Autodesk Inventor part; units mm, degrees
ref_plane "Work Plane1" through (215.9, 0, 0) normal (1, 0, 0) x (0, 0, -1)
ref_plane "YZ Plane" through (0, 0, 0) normal (1, 0, 0) x (0, 1, 0)
ref_plane "XZ Plane" through (0, 0, 0) normal (0, 1, 0) x (-1, 0, 0)
sketch "Sketch1" plane through (0, 0, 0) normal (1, 0, 0) x (0, 1, 0)
  line L0 (0, -50.8) -> (0, 50.8) construction
  line L1 (19.05, -50.8) -> (19.05, 50.8)
  line L2 (-19.05, 50.8) -> (-19.05, -50.8)
  arc A0 (-19.05, -50.8) -> (19.05, -50.8) centre (0, -50.8) ccw
  arc A1 (19.05, 50.8) -> (-19.05, 50.8) centre (0, 50.8) ccw
  circle A2 centre (0, 50.8) radius 14.2875
  circle A3 centre (0, -50.8) radius 6.35
  point P0 (0, 0)
  dimension "d0" = 50.8
  dimension "d1" = 38.1
  dimension "d2" = 28.575
  dimension "d12" = 12.7
extrude "Extrusion1" add sketch "Sketch1" along normal blind 7.9375
sketch "Sketch2" plane through (7.9375, 0, 0) normal (1, 0, 0) x (0, 0, -1)
  circle A0 centre (0, 0) radius 12.7
  circle A1 centre (0, 0) radius 15.875
  dimension "d5" = 25.4
  dimension "d6" = 31.75
extrude "Extrusion2" add sketch "Sketch2" along normal blind 207.9625
ref_plane "Work Plane1" through (215.9, 0, 0) normal (1, 0, 0) x (0, 0, -1)
sketch "Sketch3" plane through (215.9, 0, 0) normal (1, 0, 0) x (0, 0, -1)
  arc A0 (-50.8, 19.05) -> (-50.8, -19.05) centre (-50.8, 0) ccw
  circle A1 centre (-50.8, 0) radius 14.2875
  line L0 (50.8, 19.05) -> (-50.8, 19.05)
  arc A2 (50.8, -19.05) -> (50.8, 19.05) centre (50.8, 0) ccw
  line L1 (-50.8, -19.05) -> (50.8, -19.05)
  circle A3 centre (50.8, 0) radius 6.35
  point P0 (0, 0)
  dimension "d13" = 101.6
extrude "Extrusion3" add sketch "Sketch3" along normal blind 7.9375
properties part number "toggle" material "Steel, Wrought"
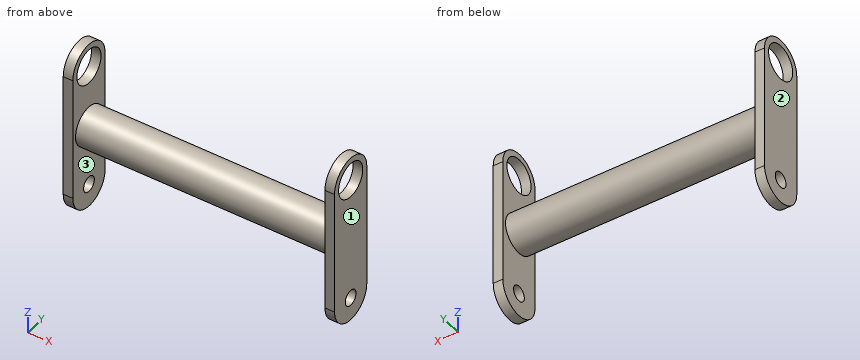
Design review of the part built by this model. Coordinates are the model's own, in mm. Face numbers are marked on the shaded views. Round coordinates to 2 decimals unless told otherwise and drop trailing zeros. Order: outer loops, then holes, each group sorted by start corner. A loop starts at its lowest first (then second) coordinate and runs counter-clockwise, first axis right, second up. Notation, with made-up numbers: (17.5, -2.5) - (64.5, -2.5) arc R10 cw to (64.5, 4.5) - close; hole circle Ø1 at (32, 78.5). An arc over 180 degrees is marked (long way). Return JSON: item names as keys, results as strings.
Q1. The part is to be moulded in two halves that separate along X. For the marked faces 1, 2 and 3, say which applies: pulls with the +X half, pulls with the -X half, needs draft (parallel to the pull), parting line crosses it, or undercut.
Computed values:
{"face 1": "pulls with the +X half", "face 2": "pulls with the -X half", "face 3": "undercut"}
Q2. Consider section A-A on y = 0. Give the number of separate pieces and of enclosed holes in the cut face, plus the area to 3 significant figures.
Computed values:
{"separate pieces": "5", "enclosed holes": "1", "area": "2,880 mm2"}
Q3. For pin 1 Ø1.5 at (x, y) = (167.5, -7.5) entering from -Z; pin 2 Ø8 at (x, y) = (46, 8.5) entering from +Z; pin 3 Ø8 at (x, y) = (28.5, -5.5) entering from -Z, all flat-tipped, find the tip position at first contact; note any pin that passes through.
Computed values:
{"pin 1": "stops at z = -14.37", "pin 2": "stops at z = 15.22", "pin 3": "stops at z = -15.8"}
Q4. Wall thickness on L1, parallel to Z at x = 5, y = 0; L2, parallel to X at y = -11, z = -63.5; L3, parallel to Y at x = 161, z = 0 (3 decimals): over which ranges is each line inside the solid? List them lowest first. Write a range as [from, to].
Computed values:
{"L1": "z = [-69.85, -57.15], [-44.45, 36.51], [65.09, 69.85]", "L2": "x = [0, 7.94], [215.9, 223.84]", "L3": "y = [-15.875, -12.7], [12.7, 15.875]"}
Q5. Consider section B-B on z = -27.5. Write out the cut boundary in (x, y).
Computed values:
{"outline": "(0, -19.05) - (7.94, -19.05) - (7.94, 19.05) - (0, 19.05) - close; (215.9, -19.05) - (223.84, -19.05) - (223.84, 19.05) - (215.9, 19.05) - close"}
Q6. Consider section D-D on x = 155. Write out the cut boundary in (y, z) (3 decimals), plus the area to 3 significant figures.
Computed values:
{"outline": "circle Ø31.75 at (0, 0); hole circle Ø25.4 at (0, 0)", "area": "285 mm2"}
